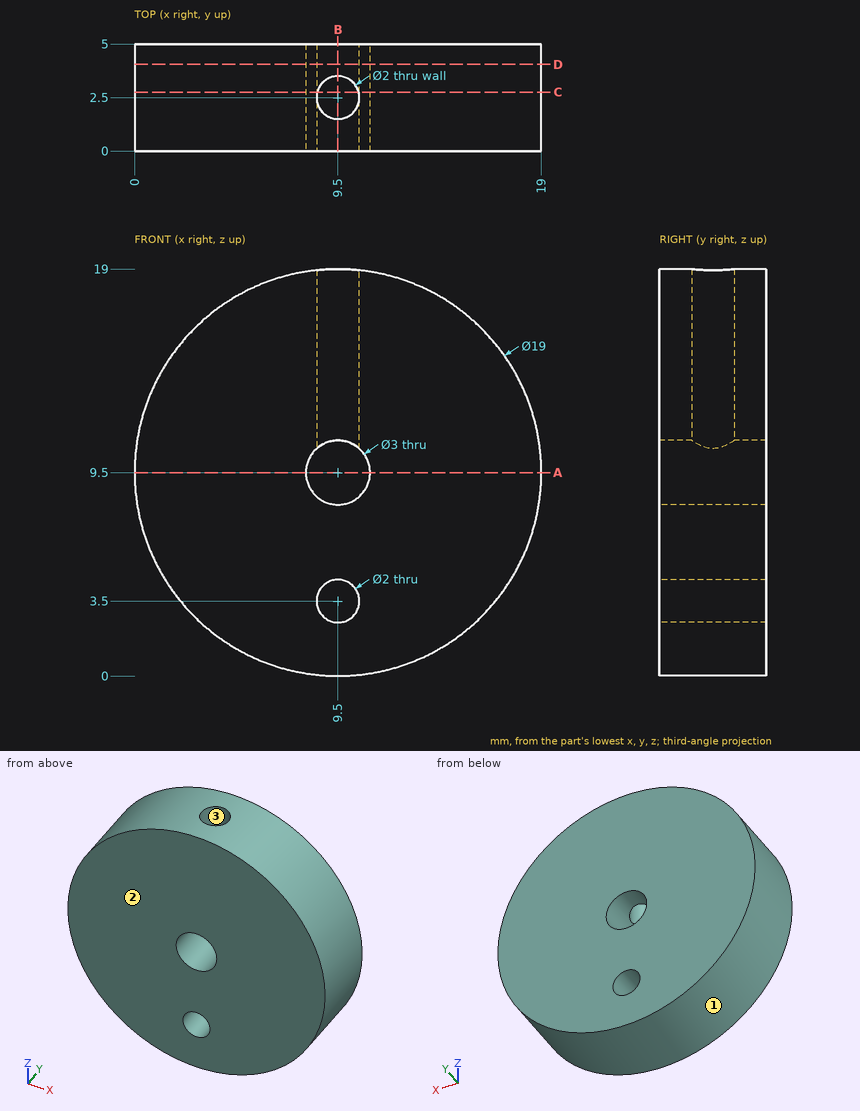
Design review of the part shown in the three views and the two pictorial views. Dimensions are in mm from the part's minimum x, y and z. Give positions to 0.01 mm unless a question says otherwise; leave off trailing zeros. Loops run counter-clockwise (first coordinate to the right, second up) from the corner with the lowest first, then second, coordinate; pieces in that order, holes last. Notation, with made-up numbers: (43.25, -9) -> (79.25, -9) arc R25 cw to (79.25, 11) -> close; hole circle Ø10 at (43.5, -2.75). An arc over 180 degrees is marked (long way). Answer as a JSON object with one key per item and string values. Group by question number.
Q1. Insertion check: pin 1 (1.6 mm diameter, centred on x = 9.5, z = 3.5, fed in from -Y); pin 2 (1.8 mm diameter, centred on x = 9.5, y = 2.5, fed in from +Z); pin 3 (1.5 mm diameter, centred on x = 16, y = 0.5, fed in from +Z); pin 4 (2 mm diameter, centred on x = 16.5, y = 3.5, fed in from +Z). Each pin has a flat end and moves straight along its axis. Give the tip position at first contact, or say it passes through.
Q2. Take a section at D-D (y = 4.05). Write out the cut boundary in (x, z).
Q3. Take a section at A-A (z = 9.5). Write out the cut boundary in (x, y), plus the area to 3 significant figures.
Q4. Take a section at B-B (x = 9.5). Write out the cut boundary in (y, z).
Q5. Draft analysis for pull direction X (two halves, no side actions). For the marked faces 1, 2 and 3, state which applies: pulls with the +X half, pulls with the -X half, needs draft (parallel to the pull), parting line crosses it, or undercut.
Q6. Wall thickness on line 1 along Z through (x, y) = (9.5, 3.8); line 2 along Z through (x, y) = (9.5, 1.8); line 3 along X through (y, z) = (3.2, 18): over which ranges is each line inside the solid? List them lowest first.
Q7. Take a section at C-C (y = 2.75). Write out the cut boundary in (x, z), plus the area to 3 significant figures.
Answer below:
{
 "1": {"pin 1": "passes through", "pin 2": "stops at z = 8.3", "pin 3": "stops at z = 17.06", "pin 4": "stops at z = 16.87"},
 "2": {"outline": "circle Ø19 at (9.5, 9.5); hole circle Ø3 at (9.5, 9.5); hole circle Ø2 at (9.5, 3.5)"},
 "3": {"outline": "(0, 0) -> (8, 0) -> (8, 5) -> (0, 5) -> close; (11, 0) -> (19, 0) -> (19, 5) -> (11, 5) -> close", "area": "80.0 mm2"},
 "4": {"outline": "(0, 0) -> (5, 0) -> (5, 2.5) -> (0, 2.5) -> close; (0, 4.5) -> (5, 4.5) -> (5, 8) -> (0, 8) -> close; (0, 11) -> (1.5, 11) -> (1.5, 19) -> (0, 19) -> close; (3.5, 11) -> (5, 11) -> (5, 19) -> (3.5, 19) -> close"},
 "5": {"face 1": "parting line crosses it", "face 2": "needs draft", "face 3": "undercut"},
 "6": {"line 1": "z = 0 to 2.5, 4.5 to 8, 11 to 19", "line 2": "z = 0 to 2.5, 4.5 to 8", "line 3": "x = 5.26 to 8.79, 10.21 to 13.74"},
 "7": {"outline": "(8.53, 10.65) -> (8.53, 18.95) arc R9.5 ccw (long way) to (10.47, 18.95) -> (10.47, 10.65) arc R1.5 cw (long way) to start; hole circle Ø2 at (9.5, 3.5)", "area": "258 mm2"}
}
